```python
from build123d import *

# Parameters (mm, degrees)
SKETCH_1_R      = 5.75
EXTRUDE_1_DEPTH = 6
SKETCH_2_R      = 6.5
EXTRUDE_2_DEPTH = 1.5
EXTRUDE_START   = -6
SKETCH_3_W      = 3
SKETCH_3_H      = 3
EXTRUDE_3_DEPTH = 12.5
SKETCH_4_W      = 12.5
SKETCH_4_H      = 12.5
EXTRUDE_4_DEPTH = 3.5


with BuildPart() as part:
    # Эскиз1 → Бобышка-Вытянуть1 (new body)
    with BuildSketch(Plane(origin=(0, 0, 0), x_dir=(1, 0, 0), z_dir=(0, 1, 0))):
        Circle(SKETCH_1_R)
    extrude(amount=EXTRUDE_1_DEPTH)

    # Эскиз2 → Бобышка-Вытянуть2 (add)
    with BuildSketch(Plane.XZ):
        Circle(SKETCH_2_R)
    extrude(amount=-EXTRUDE_2_DEPTH)

    # Эскиз3 → Бобышка-Вытянуть3 (add)
    with BuildSketch(Plane.XZ.offset(EXTRUDE_START)):
        Rectangle(SKETCH_3_W, SKETCH_3_H)
    extrude(amount=EXTRUDE_3_DEPTH)

    # Эскиз4 → Бобышка-Вытянуть4 (add)
    with BuildSketch(Plane.XZ.offset(6.5)):
        Rectangle(SKETCH_4_W, SKETCH_4_H)
    extrude(amount=-EXTRUDE_4_DEPTH)


solid = part.part
```
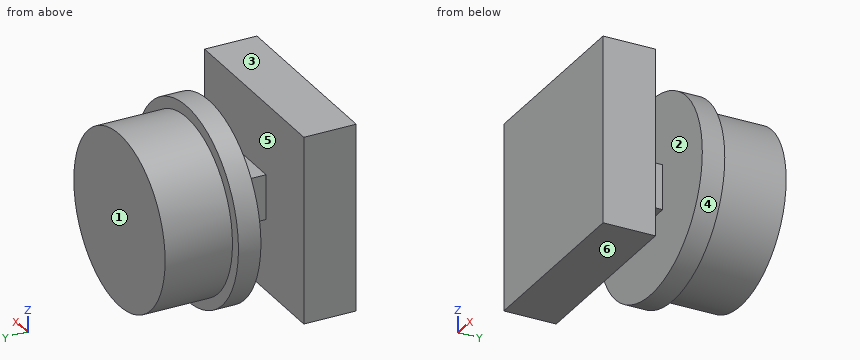
CAD build for the part. Positions are in the model's coordinates, mm. Face numbers are marked on the shaded views. A direction names the side the tool comes from. Round coordinates to 2 decimals unless told otherwise and drop trailing zeros. Write each loop counter-clockwise with the first axis right and the second up, starting at its lowest first coordinate (ties: lowest second). Pieces come first, ordered by that corner, then holes. Notation, with made-up numbers: M 10,-31.75 L 19,-31.75 A24 cw 19,-2.75 Z; hole C 3.5,40 d11. An arc over 180 degrees is marked long. One line per question, with ' | ' between items.
1. Cut at D-D on y = -2.75. Write the cut outline in (x, z), and give its area (3 significant figures).
Working result:
outline: M -1.5,-1.5 L 1.5,-1.5 L 1.5,1.5 L -1.5,1.5 Z | area: 9.00 mm2
2. Cut at C-C on z = 0. Write the cut outline in (x, y).
Working result:
outline: M -6.5,0 L -1.5,0 L -1.5,-3 L -6.25,-3 L -6.25,-6.5 L 6.25,-6.5 L 6.25,-3 L 1.5,-3 L 1.5,0 L 6.5,0 L 6.5,1.5 L 5.75,1.5 L 5.75,6 L -5.75,6 L -5.75,1.5 L -6.5,1.5 Z
3. Cut at A-A on x = 4.5. Write the cut outline in (y, z), and give its area (3 significant figures).
Working result:
outline: M -6.5,-6.25 L -3,-6.25 L -3,6.25 L -6.5,6.25 Z; M 0,-4.69 L 1.5,-4.69 L 1.5,-3.58 L 6,-3.58 L 6,3.58 L 1.5,3.58 L 1.5,4.69 L 0,4.69 Z | area: 90.0 mm2
4. Mould opens along Y. For the marked faces 1, 2 and 3 say: pulls with the +Y half, pulls with the -Y half, needs draft (parallel to the pull), parting line crosses it, or undercut.
Working result:
face 1: pulls with the +Y half | face 2: undercut | face 3: needs draft
5. Which spindle directions (+Z, -Z, +X, -X, +Y, -Y) get a long thin tool onto all of the face, cutting with end or side? Do the marked faces 4, 5 and 6. Say none if no direction does.
Working result:
face 4: +Y | face 5: none | face 6: -Z, +X, -X, -Y
6. Probe L1, parallel to Y at x = 2, z = 5.25; L2, parallel to Y at x = 5.75, z = 1.25; L3, parallel to X at y = -3.25, z = -4.5. List the from-to ranges inside material, lowest first. Write a range as from..to.
Working result:
L1: -6.5..-3, 0..6 | L2: -6.5..-3, 0..1.5 | L3: -6.25..6.25
7. Cut at B-B on z = -4.5. Write the cut outline in (x, y).
Working result:
outline: M -6.25,-6.5 L 6.25,-6.5 L 6.25,-3 L -6.25,-3 Z; M -4.69,0 L 4.69,0 L 4.69,1.5 L 3.58,1.5 L 3.58,6 L -3.58,6 L -3.58,1.5 L -4.69,1.5 Z
8. Pin check, flat tips, straight feed: pin 1 Ø1.8 at (x, y) = (0.5, -4) entering from +Z; pin 2 Ø2.5 at (x, y) = (0.5, -1.5) entering from -Z; pin 3 Ø1 at (y, z) = (2.5, 4) entering from -X. Stop position of each tip, or through.
Working result:
pin 1: z = 6.25 | pin 2: z = -1.5 | pin 3: x = -4.56
